Check sheet for the modelled part. Datum: model origin and axes. Units: mm. A direction names the side the tool comes from. Give positions to 0.01 mm unless a question says otherwise; leave off trailing zeros. Loops run counter-clockwise (first coordinate to the right, second up) from the corner with the lowest first, then second, coordinate; pieces in that order, holes last. Notation, with made-up numbers: (-9.75, 31) -> (24.25, 31) arc R26 cw to (24.25, 59) -> close; hole circle Ø5 at (5.25, 77.5). An arc over 180 degrees is marked (long way). Write each question's results on one line, items separated by ' | '. Start each with the question number.
1. Cross-section at A-A on z = 33.5. Record the boundary of the cut face in (x, y), and give its area (3 significant figures).
2. Material ranges on L1, parallel to Y at x = 45.75, z = 7.5; L2, parallel to Y at x = -45.75, z = 10.75, recorded low to high. Write a range as from..to.
3. Cross-section at C-C on y = -45.75. Record the boundary of the cut face in (x, z).
4. Cross-section at B-B on x = 24. Record the boundary of the cut face in (y, z).
5. Cross-section at D-D on z = 8. Record the boundary of the cut face in (x, y), and give its area (3 significant figures).
6. Tool access check on faces 4 (the face through (-45.64, -38.49, 17.85)), 5 (the face through (46, 41.5, 110)), 6 (the face through (38.65, 45.48, 94.99)), 7 (the face through (46, 41.5, 4)). Record the directions out of +Z, -Z, +X, -X, +Y, -Y that give a thin tool (end or side, any length) a straight path to the whole face; none if there is none.
7. Mould release check, pull along X, two halves, no side actions. Record for faces 1 (the face through (38.49, -38.65, 10.86)), 2 (the face through (-45, 45, 113.5)), 3 (the face through (38.65, -45.64, 94.99)): +X half, -X half, draft (parallel to the pull), parting line (faces both ways), or undercut.
8. Gauge pin test, flat ends, axial feed: pin 1 Ø10 at (x, y) = (-10.5, 40) entering from +Z; pin 2 Ø2.5 at (x, y) = (15.5, -47.5) entering from -Z; pin 3 Ø8 at (y, z) = (-34, 50.5) entering from -X. Record the tip position at first contact, or that the pin passes through.
from build123d import *

# Parameters (mm, degrees)
F0_W      = 100
F0_H      = 100
F1_DEPTH  = 113.5
F3_DEPTH  = 25
F4_DEPTH  = 120
F5_W      = 83
F5_H      = 6.5
F5_H_2    = 7
F6_DEPTH  = 105
F7_W      = 83
F7_H      = 7
F7_H_2    = 6.5
F8_DEPTH  = 105
F9_DEPTH  = 1
F10_R     = 1
F11_R     = 2.5
F12_DEPTH = 19


with BuildPart() as f1:
    # F0 (on Top) → F1 (new body)
    with BuildSketch(Plane.XY):
        Rectangle(F0_W, F0_H)
    extrude(amount=F1_DEPTH)

    # F2 (on Top) → F3 (join)
    with BuildSketch(Plane.XY):
        with BuildLine():
            Line((31.5, 41.5), (-31.5, 41.5))
            ThreePointArc((-31.5, 41.5), (-38.5710678119, 38.5710678119), (-41.5, 31.5))
            Line((-41.5, 31.5), (-41.5, -31.5))
            ThreePointArc((-41.5, -31.5), (-38.5710678119, -38.5710678119), (-31.5, -41.5))
            Line((-31.5, -41.5), (31.5, -41.5))
            ThreePointArc((31.5, -41.5), (38.5710678119, -38.5710678119), (41.5, -31.5))
            Line((41.5, -31.5), (41.5, 31.5))
            ThreePointArc((41.5, 31.5), (38.5710678119, 38.5710678119), (31.5, 41.5))
        make_face()
    extrude(amount=F3_DEPTH)

    # F2 (on Top) → F4 (cut)
    with BuildSketch(Plane.XY):
        with BuildLine():
            Line((31.5, 41.5), (-31.5, 41.5))
            ThreePointArc((-31.5, 41.5), (-38.5710678119, 38.5710678119), (-41.5, 31.5))
            Line((-41.5, 31.5), (-41.5, -31.5))
            ThreePointArc((-41.5, -31.5), (-38.5710678119, -38.5710678119), (-31.5, -41.5))
            Line((-31.5, -41.5), (31.5, -41.5))
            ThreePointArc((31.5, -41.5), (38.5710678119, -38.5710678119), (41.5, -31.5))
            Line((41.5, -31.5), (41.5, 31.5))
            ThreePointArc((41.5, 31.5), (38.5710678119, 38.5710678119), (31.5, 41.5))
        make_face()
    extrude(amount=F4_DEPTH, mode=Mode.SUBTRACT)

    # F5 (on face) → F6 (cut)
    with BuildSketch(Plane(origin=(-50, 0, 0), x_dir=(0, -1, 0), z_dir=(-1, 0, 0))):
        with BuildLine():
            ThreePointArc((-41.5, 25), (-38.5710678119, 17.9289321881), (-31.5, 15))
            Line((-31.5, 15), (31.5, 15))
            ThreePointArc((31.5, 15), (38.5710678119, 17.9289321881), (41.5, 25))
            Line((41.5, 25), (41.5, 88))
            ThreePointArc((41.5, 88), (38.5710678119, 95.0710678119), (31.5, 98))
            Line((31.5, 98), (-31.5, 98))
            ThreePointArc((-31.5, 98), (-38.5710678119, 95.0710678119), (-41.5, 88))
            Line((-41.5, 88), (-41.5, 25))
        make_face()
        with Locations((0, 3.25)):
            Rectangle(F5_W, F5_H)
        with Locations((0, 110)):
            Rectangle(F5_W, F5_H_2)
    extrude(amount=-F6_DEPTH, mode=Mode.SUBTRACT)

    # F7 (on face) → F8 (cut)
    with BuildSketch(Plane.XZ.offset(50)):
        with Locations((0, 110)):
            Rectangle(F7_W, F7_H)
        with BuildLine():
            ThreePointArc((-31.5, 98), (-38.5710678119, 95.0710678119), (-41.5, 88))
            Line((-41.5, 88), (-41.5, 25))
            ThreePointArc((-41.5, 25), (-38.5710678119, 17.9289321881), (-31.5, 15))
            Line((-31.5, 15), (31.5, 15))
            ThreePointArc((31.5, 15), (38.5710678119, 17.9289321881), (41.5, 25))
            Line((41.5, 25), (41.5, 88))
            ThreePointArc((41.5, 88), (38.5710678119, 95.0710678119), (31.5, 98))
            Line((31.5, 98), (-31.5, 98))
        make_face()
        with Locations((0, 3.25)):
            Rectangle(F7_W, F7_H_2)
    extrude(amount=-F8_DEPTH, mode=Mode.SUBTRACT)

    # F9 (cut): faces of the model
    f9_faces = [f1.faces().sort_by_distance(p)[0] for p in [
        (-45.75, -45.75, 0),
        (-45.75, -45.75, 113.5),
        (45.75, 45.75, 113.5),
        (45.75, 45.75, 0),
    ]]
    extrude(f9_faces, amount=-F9_DEPTH, dir=(0, 0, -1), mode=Mode.SUBTRACT)

    # F10
    f10_edges = [f1.edges().sort_by_distance(p)[0] for p in [
        (45.75, -50, 0),
        (50, -45.75, 0),
        (50, -45.75, 113.5),
        (45.75, -50, 113.5),
        (50, 45.75, 113.5),
        (45.75, 50, 113.5),
        (50, 45.75, 1),
        (45.75, 50, 1),
        (-45.75, 50, 0),
        (-50, 45.75, 0),
        (-50, -45.75, 1),
        (-45.75, -50, 1),
        (-50, -45.75, 113.5),
        (-45.75, -50, 113.5),
        (-50, 45.75, 113.5),
        (-45.75, 50, 113.5),
    ]]
    fillet(f10_edges, radius=F10_R)

    # F11 (on face) → F12 (cut)
    with BuildSketch(Plane(origin=(0, 0, 1), x_dir=(1, 0, 0), z_dir=(0, 0, -1))):
        with Locations((-45.75, 45.75)):
            Circle(F11_R)
        with Locations((45.75, -45.75)):
            Circle(F11_R)
    extrude(amount=-F12_DEPTH, mode=Mode.SUBTRACT)


solid = f1.part
Geometry says:
1) outline: (-50, -50) -> (-41.5, -50) -> (-41.5, -41.5) -> (-50, -41.5) -> close; (-50, 41.5) -> (-41.5, 41.5) -> (-41.5, 50) -> (-50, 50) -> close; (41.5, -50) -> (50, -50) -> (50, -41.5) -> (41.5, -41.5) -> close; (41.5, 41.5) -> (50, 41.5) -> (50, 50) -> (41.5, 50) -> close | area: 289 mm^2
2) L1: -50..43.25, 48.25..50 | L2: -50..-48.25, -43.25..50
3) outline: (-50, 2) arc R1 ccw to (-49, 1) -> (-48.25, 1) -> (-48.25, 20) -> (-43.25, 20) -> (-43.25, 1) -> (-41.5, 1) -> (-41.5, 6.5) -> (41.5, 6.5) -> (41.5, 0) -> (49, 0) arc R1 ccw to (50, 1) -> (50, 112.5) arc R1 ccw to (49, 113.5) -> (41.5, 113.5) -> (41.5, 106.5) -> (-41.5, 106.5) -> (-41.5, 113.5) -> (-49, 113.5) arc R1 ccw to (-50, 112.5) -> close; hole (-41.5, 25) arc R10 ccw to (-31.5, 15) -> (31.5, 15) arc R10 ccw to (41.5, 25) -> (41.5, 88) arc R10 ccw to (31.5, 98) -> (-31.5, 98) arc R10 ccw to (-41.5, 88) -> close
4) outline: (-50, 6.5) -> (-41.5, 6.5) -> (-41.5, 15) -> (-50, 15) -> close; (-50, 98) -> (-41.5, 98) -> (-41.5, 106.5) -> (-50, 106.5) -> close; (41.5, 6.5) -> (50, 6.5) -> (50, 15) -> (41.5, 15) -> close; (41.5, 98) -> (50, 98) -> (50, 106.5) -> (41.5, 106.5) -> close
5) outline: (-50, -50) -> (50, -50) -> (50, 50) -> (-50, 50) -> close; hole circle Ø5 at (-45.75, -45.75); hole (-41.5, -31.5) arc R10 ccw to (-31.5, -41.5) -> (31.5, -41.5) arc R10 ccw to (41.5, -31.5) -> (41.5, 31.5) arc R10 ccw to (31.5, 41.5) -> (-31.5, 41.5) arc R10 ccw to (-41.5, 31.5) -> close; hole circle Ø5 at (45.75, 45.75) | area: 3,160 mm^2
6) face 4: +X, -X | face 5: +Z, +X, -X | face 6: +Y, -Y | face 7: -Z, +X, -X
7) face 1: undercut | face 2: draft | face 3: undercut
8) pin 1: z = 106.5 | pin 2: z = 6.5 | pin 3: through
